Read the model definition and answer for the solid it produces. Units are mm, in the model's axes. Face numbers are marked on the shaded views. A direction names the side the tool comes from. Round coordinates to 2 decimals unless told otherwise and drop trailing zeros. Write each loop counter-clockwise with the first axis right and the second up, starting at its lowest first coordinate (ties: lowest second). Pieces come first, ordered by that corner, then holes. Notation, with made-up numbers: (-34.75, 18.25) - (4.25, 18.25) arc R19 ccw to (4.25, 24.25) - close; hole circle Ø7 at (12.25, 57). An arc over 180 degrees is marked (long way). One line per item, written item: value. Start each with the question number.
(1) The mould has two halves that part along Y. Classify the marked faces 1, 2 and 3: +Y half, -Y half, draft (parallel to the pull), parting line (faces both ways), or undercut.
(2) For the marked faces 4 and 5, determine the directions among +Z, -Z, +X, -X, +Y, -Y from which every point of the face is accessible in a straight line to the end or side of a thin tool.
(3) Find the intervals of material crossed by L1, parallel to Y at x = 183, z = 12.75; L2, parallel to Z at x = 68, y = 11.5, in increasing order.
(4) Flat-ended cylindrical pins translate along their axes: pin 1 Ø8 at (y, z) = (23, 2) entering from -X; pin 2 Ø12.5 at (x, y) = (70, 16.5) entering from +Z. Find the tip coordinate at first contact, or state that the pin passes through.
(5) A cutting plane is placed at A-A, the plane z = 10.5. State how many separate pieces and enclosed holes the cut face has, plus the area to 3 significant figures.
(6) A cutting plane is placed at C-C, the plane x = 170.5. Determine the outline of the cut face in (y, z), plus the area to 3 significant figures.
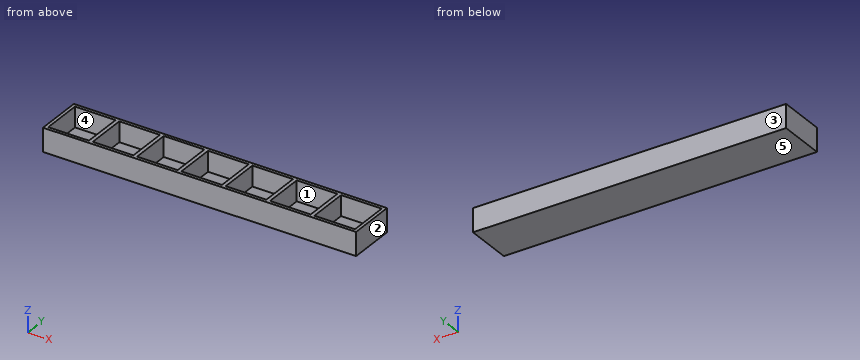
from build123d import *

# Parameters (mm, degrees)
SKETCH_W            = 195.8
SKETCH_H            = 29.4
PAD_DEPTH           = 14.7
SKETCH001_W         = 25.4
SKETCH001_H         = 25.4
POCKET_DEPTH        = 12.7
LINEARPATTERN_COUNT = 7
LINEARPATTERN_PITCH = 27.733333


with BuildPart() as part:
    # Sketch → Pad (new body)
    with BuildSketch(Plane.XY):
        with Locations((97.9, 14.7)):
            Rectangle(SKETCH_W, SKETCH_H)
    extrude(amount=PAD_DEPTH)

    # Sketch001 → Pocket (cut)
    with BuildSketch(Plane.XY.offset(14.7)):
        with Locations((14.7, 14.7)):
            Rectangle(SKETCH001_W, SKETCH001_H)
    pocket = extrude(amount=-POCKET_DEPTH, mode=Mode.SUBTRACT)

    # LinearPattern: Pocket ×7
    with Locations(*[(i * LINEARPATTERN_PITCH, 0, 0) for i in range(1, LINEARPATTERN_COUNT)]):
        add(pocket, mode=Mode.SUBTRACT)


solid = part.part
Here are the results:
1. face 1: undercut
1. face 2: draft
1. face 3: +Y half
2. face 4: +Z
2. face 5: -Z, +X, -X, +Y, -Y
3. L1: 0 to 2, 27.4 to 29.4
3. L2: 0 to 2
4. pin 1: x = 0
4. pin 2: z = 2
5. separate pieces: 1
5. enclosed holes: 7
5. area: 1,240 mm²
6. outline: (0, 0) - (29.4, 0) - (29.4, 14.7) - (27.4, 14.7) - (27.4, 2) - (2, 2) - (2, 14.7) - (0, 14.7) - close
6. area: 110 mm²
